The listing builds one solid part. Answer for the finished solid, in the listing's coordinates (mm). Face numbers are marked on the shaded views. A direction names the side the tool comes from. Coordinates: 2 decimals unless noted, no trailing zeros. Order: outer loops, then holes, each group sorted by start corner. A loop starts at its lowest first (then second) coordinate and runs counter-clockwise, first axis right, second up. Notation, with made-up numbers: (60, 35.5) -> (104, 35.5) arc R16 cw to (104, 49.5) -> close; hole circle Ø5 at (-11.75, 2). An arc over 180 degrees is marked (long way). Return JSON: item names as keys, results as strings.
Autodesk Inventor part; units mm, degrees
ref_plane "YZ Plane" through (0, 0, 0) normal (1, 0, 0) x (0, 1, 0)
ref_plane "XZ Plane" through (0, 0, 0) normal (0, 1, 0) x (-1, 0, 0)
ref_plane "XY Plane" through (0, 0, 0) normal (0, 0, 1) x (1, 0, 0)
sketch "Skizze1" plane through (0, 0, 0) normal (1, 0, 0) x (0, 1, 0)
  arc A0 (12.9164, -2.8566) -> (12.4836, 2.9608) centre (12, 0) ccw
  line L0 (12.9164, -2.8566) -> (0, -7)
  line L1 (0, -7) -> (0, 5)
  line L2 (0, 5) -> (12.4836, 2.9608)
  point P0 (0, 0)
  dimension "d0" = 3
  dimension "d1" = 12
  dimension "d2" = 12
  dimension "d3" = 5
extrude "Extrusion1" add sketch "Skizze1" along normal mid plane 2
sketch "Skizze2" plane through (0, 0, 0) normal (0, 1, 0) x (-1, 0, 0)
  line L0 (-1, 2.9608) -> (-1, 5)
  line L1 (-1, 5) -> (4, 5)
  line L2 (4, 5) -> (4, -7)
  line L3 (4, -7) -> (-1, -7)
  line L4 (-1, -7) -> (-1, 5)
  line L5 (1, -7) -> (-1, -7)
  point P0 (0, 0)
  dimension "d6" = 5
extrude "Extrusion2" add sketch "Skizze2" against normal blind 3
fillet "Rundung1" radius 2 1 edges at (-1, 0, -1)
sketch "Skizze3" plane through (1, 0, 0) normal (1, 0, 0) x (0, 0, -1)
  arc A0 (2.8566, 12.9164) -> (-2.9608, 12.4836) centre (0, 12) ccw
  circle A1 centre (0, 12) radius 0.7
  line L0 (0, 12) -> (0, -3) construction
  line L1 (7, -3) -> (-5, -3)
  circle A2 centre (0, 8) radius 0.7
  point P0 (0, 0)
  dimension "d10" = 1.4
  dimension "d13" = 4
extrude "Extrusion3" cut sketch "Skizze3" against normal blind 4.75
fillet "Rundung2" radius 2 4 edges at (-4, -1.5, 5) (1, -1.5, 5) (1, -1.5, -7) (-4, -1.5, -7)
properties part number "P_Wing_aileron_lever"
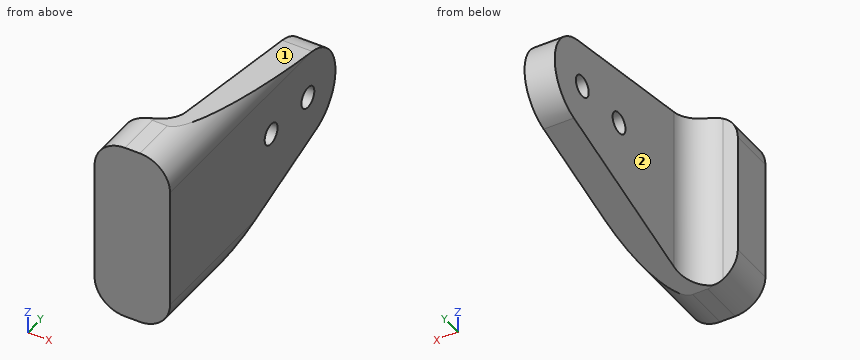
1. Each of these flat-tipped pins is pushed along its axis until it touches: pin 1 Ø3.5 at (y, z) = (11, -1) entering from -X; pin 2 Ø2 at (x, z) = (-1.5, -1) entering from +Y. Where does it stop, or does it pass through?
Answer block:
{"pin 1": "stops at x = -1", "pin 2": "stops at y = 15"}
2. The part is cut by section C-C on x = 0.05. Give the vertices of the cut face in (y, z).
Answer block:
{"outline": "(-3, -6.7) -> (0.93, -6.7) -> (12.92, -2.86) arc R3 ccw to (12.48, 2.96) -> (1.82, 4.7) -> (-3, 4.7) -> close; hole circle Ø1.4 at (8, 0); hole circle Ø1.4 at (12, 0)"}
3. The part is cut by section B-B on y = 11.75. Give the vertices of the cut face in (x, z), and give its area (3 significant figures).
Answer block:
{"outline": "(-1, -3.23) -> (1, -3.23) -> (1, -0.65) -> (-1, -0.65) -> close; (-1, 0.65) -> (1, 0.65) -> (1, 3) arc R2 ccw to (1, 3.08) -> (-1, 3.08) -> close", "area": "10.0 mm2"}
4. For the marked faces 1 and 2, determine the directions among +Z, -Z, +X, -X, +Y, -Y from which every point of the face is accessible in a straight line to the end or side of a thin tool.
Answer block:
{"face 1": "+Z, +X, -X, +Y", "face 2": "+Z, -Z, -X, +Y"}
5. The part is cut by section D-D on z = -4. Give the vertices of the cut face in (x, y).
Answer block:
{"outline": "(-4, -3) -> (1, -3) -> (1, 9.35) -> (-1, 9.35) -> (-1, 2) arc R2 cw to (-3, 0) -> (-4, 0) -> close"}
6. Consider line 1 (Y direction, x = 0.4, z = 0); line 2 (Y direction, x = -2.95, z = 4); line 3 (X direction, y = 5.5, z = 1.5). Determine where each line is inside the solid, lowest interval first. Write a range as from..to.
Answer block:
{"line 1": "y = -3..7.3, 8.7..11.3, 12.7..15", "line 2": "y = -3..0", "line 3": "x = -1..1"}
7. The part is cut by section A-A on z = 0. Give the vertices of the cut face in (x, y).
Answer block:
{"outline": "(-4, -3) -> (1, -3) -> (1, 7.3) -> (-1, 7.3) -> (-1, 2) arc R2 cw to (-3, 0) -> (-4, 0) -> close; (-1, 8.7) -> (1, 8.7) -> (1, 11.3) -> (-1, 11.3) -> close; (-1, 12.7) -> (1, 12.7) -> (1, 15) -> (-1, 15) -> close"}
